Build history of the part. All positions in model axes, mm. Give positions to 0.01 mm unless a question says otherwise; leave off trailing zeros. Order: outer loops, then holes, each group sorted by start corner. A loop starts at its lowest first (then second) coordinate and runs counter-clockwise, first axis right, second up. Notation, with made-up numbers: M 69,9.25 L 81,9.25 A30 ccw 81,42.25 Z; hole C 71.5,-37.5 d4. An arc over 180 degrees is marked long. One line per item, written item: value.
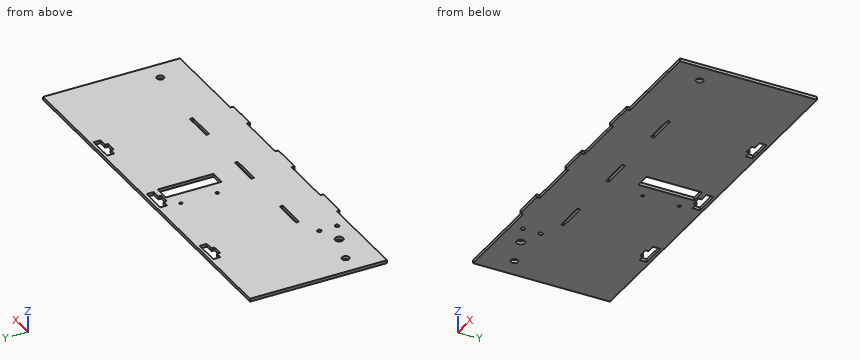
from build123d import *

# Parameters (mm, degrees)
CROQUIS1_R              = 1.5
CROQUIS1_R_2            = 3.5
CROQUIS1_R_3            = 4
CROQUIS1_R_4            = 2
CROQUIS1_W              = 30
CROQUIS1_H              = 3
CROQUIS1_W_2            = 15
CROQUIS1_H_2            = 55
SALIENTE_EXTRUIR4_DEPTH = 3


with BuildPart() as part:
    # Croquis1 → Saliente-Extruir4 (new body)
    with BuildSketch(Plane.XY):
        Polygon((-190, -67.5), (-97.5, -67.5), (-97.5, -70.5), (-67.5, -70.5), (-67.5, -67.5), (-15, -67.5), (-15, -70.5), (15, -70.5), (15, -67.5), (67.5, -67.5), (67.5, -70.5), (97.5, -70.5), (97.5, -67.5), (190, -67.5), (190, 67.5), (-190, 67.5), align=None)
        with Locations((-22, 45.5)):
            Circle(CROQUIS1_R, mode=Mode.SUBTRACT)
        with Locations((-22, 9.5)):
            Circle(CROQUIS1_R, mode=Mode.SUBTRACT)
        with Locations((-170, -37.5)):
            Circle(CROQUIS1_R_2, mode=Mode.SUBTRACT)
        with Locations((-139.5, -47.5)):
            Circle(CROQUIS1_R_3, mode=Mode.SUBTRACT)
        with Locations((-119.3, -38.75)):
            Circle(CROQUIS1_R_4, mode=Mode.SUBTRACT)
        with Locations((-119.3, -56.25)):
            Circle(CROQUIS1_R_4, mode=Mode.SUBTRACT)
        with Locations((170, -37.5)):
            Circle(CROQUIS1_R_2, mode=Mode.SUBTRACT)
        with Locations((82.5, -29)):
            Rectangle(CROQUIS1_W, CROQUIS1_H, mode=Mode.SUBTRACT)
        with Locations((0, -29)):
            Rectangle(CROQUIS1_W, CROQUIS1_H, mode=Mode.SUBTRACT)
        with Locations((-82.5, -29)):
            Rectangle(CROQUIS1_W, CROQUIS1_H, mode=Mode.SUBTRACT)
        Polygon((-19.6, 64.5), (-19.6, 57.5), (-13, 57.5), (-13, 54.5), (-3, 54.5), (-3, 57.5), (5.4, 57.5), (5.4, 64.5), align=None, mode=Mode.SUBTRACT)
        Polygon((-117.1, 64.5), (-117.1, 57.5), (-110.5, 57.5), (-110.5, 54.5), (-100.5, 54.5), (-100.5, 57.5), (-92.1, 57.5), (-92.1, 64.5), align=None, mode=Mode.SUBTRACT)
        Polygon((77.9, 64.5), (77.9, 57.5), (84.5, 57.5), (84.5, 54.5), (94.5, 54.5), (94.5, 57.5), (102.9, 57.5), (102.9, 64.5), align=None, mode=Mode.SUBTRACT)
        with Locations((0, 25)):
            Rectangle(CROQUIS1_W_2, CROQUIS1_H_2, mode=Mode.SUBTRACT)
    extrude(amount=SALIENTE_EXTRUIR4_DEPTH)


solid = part.part
1) Saw through at B-B, the plane y = -47.5. Write the cut outline in (x, z), then the cut area to 3 significant figures.
Check values:
outline: M -190,0 L -143.5,0 L -143.5,3 L -190,3 Z; M -135.5,0 L 190,0 L 190,3 L -135.5,3 Z
area: 1,120 mm^2
2) Saw through at D-D, the plane x = 118.5. Write the cut outline in (y, z).
Check values:
outline: M -67.5,0 L 67.5,0 L 67.5,3 L -67.5,3 Z
3) Drill centre lines: probe 1 along Y at (x, z) = (-22, 1); probe 2 along Y at (x, z) = (-119.3, 1.7); probe 3 along X at (y, z) = (59.5, 1.2). Where is each one in solid material? Low to high. Write a range as from..to.
Check values:
probe 1: -67.5..8, 11..44, 47..67.5
probe 2: -67.5..-58.25, -54.25..-40.75, -36.75..67.5
probe 3: -190..-117.1, -92.1..-19.6, 5.4..77.9, 102.9..190
4) Pin check, flat tips, straight feed: pin 1 (1.5 mm diameter, centred on y = -69, z = 1.5, fed in from -X); pin 2 (1.5 mm diameter, centred on x = -144, z = 0.5, fed in from -Y). Stop position of each tip, or through.
Check values:
pin 1: x = -97.5
pin 2: y = -67.5
5) Saw through at C-C, the plane z = 1.55. Give the number of separate pieces and of enclosed holes in the cut face, then the cut area to 3 significant figures.
Check values:
separate pieces: 1
enclosed holes: 14
area: 49,700 mm^2
6) Saw through at A-A, the plane x = -170. Write the cut outline in (y, z), then the cut area to 3 significant figures.
Check values:
outline: M -67.5,0 L -41,0 L -41,3 L -67.5,3 Z; M -34,0 L 67.5,0 L 67.5,3 L -34,3 Z
area: 384 mm^2
